Check sheet for the modelled part. Datum: model origin and axes. Units: mm. Round coordinates to 2 decimals unless told otherwise and drop trailing zeros. Loops run counter-clockwise (first coordinate to the right, second up) from the corner with the lowest first, then second, coordinate; pieces in that order, holes last. Notation, with made-up numbers: (38, 25.25) - (42, 25.25) arc R12 ccw to (42, 32.25) - close; hole circle Ø4 at (25, 80). An arc over 180 degrees is marked (long way). Answer in a Markdown table with one row per item. Add a question column.
(1) Mould release check, pull along X, two halves, no side actions. Record for faces 1 (the cylindrical face through (-1.38, 0.07, 6.2)), 2 (the flat face through (21.997, 0, 0)), 3 (the conical face through (-0.056, -4.522, -22.824)): +X half, -X half, draft (parallel to the pull), parting line (faces both ways), or undercut.
(2) Thickness scan on line 1 along Z through (x, y) = (0, -2); line 2 along Z through (x, y) = (1, 2); line 3 along X through (y, z) = (2.5, 0.5). Record the ranges inside material, lowest first.
(3) Gauge pin test, flat ends, axial feed: pin 1 (1 mm diameter, centred on x = -12.5, y = 2, fed in from +Z); pin 2 (1.5 mm diameter, centred on y = -1.5, z = 17.5, fed in from +X); pin 3 (10 mm diameter, centred on x = 0, z = 0, fed in from -Y); pin 4 (3 mm diameter, centred on x = 16.5, y = 0, fed in from +Z). Record the tip position at first contact, or that the pin passes through.
(4) Cross-section at A-A on y = 2. Enter the section's corners in (x, z), then the cut area to 3 significant figures.
from build123d import *

# Parameters (mm, degrees)
BOSS_EXTRUDE1_DEPTH = 5
SKETCH2_R           = 6.35
CUT_EXTRUDE1_DEPTH  = 11
SKETCH3_OUTSIDE_W   = 97.688
SKETCH3_OUTSIDE_H   = 104.494
SKETCH3_OUTSIDE_R   = 21.997045256
CUT_EXTRUDE2_DEPTH  = 11
CUT_EXTRUDE2_TAPER  = 60


with BuildPart() as part:
    # Sketch1 → Boss-Extrude1 (new body, symmetric)
    with BuildSketch(Plane(origin=(0, 0, 0), x_dir=(1, 0, 0), z_dir=(0, 1, 0))):
        Polygon((21.997045256, 12.7), (0, 25.4), (-21.997045256, 12.7), (-21.997045256, -12.7), (0, -25.4), (21.997045256, -12.7), align=None)
    extrude(amount=BOSS_EXTRUDE1_DEPTH, both=True)

    # Sketch2 → Cut-Extrude1 (cut, through all)
    with BuildSketch(Plane(origin=(0, 5, 0), x_dir=(1, 0, 0), z_dir=(0, 1, 0))):
        Circle(SKETCH2_R)
    extrude(amount=-CUT_EXTRUDE1_DEPTH, mode=Mode.SUBTRACT)

    # Sketch3 outside → Cut-Extrude2 (cut, through all)
    with BuildSketch(Plane(origin=(0, 5, 0), x_dir=(1, 0, 0), z_dir=(0, 1, 0))):
        Rectangle(SKETCH3_OUTSIDE_W, SKETCH3_OUTSIDE_H)
        Circle(SKETCH3_OUTSIDE_R, mode=Mode.SUBTRACT)
    cut_extrude2 = extrude(amount=-CUT_EXTRUDE2_DEPTH, taper=CUT_EXTRUDE2_TAPER, mode=Mode.SUBTRACT)

    # Mirror1: Cut-Extrude2 across plane
    add(cut_extrude2.mirror(Plane.ZX), mode=Mode.SUBTRACT)


solid = part.part
Answers:
| question | item | result |
|---|---|---|
| 1 | face 1 | undercut |
| 1 | face 2 | +X half |
| 1 | face 3 | parting line |
| 2 | line 1 | z = -25.4 to -6.35, 6.35 to 25.4 |
| 2 | line 2 | z = -24.82 to -6.27, 6.27 to 24.82 |
| 2 | line 3 | x = -22 to -6.33, 6.33 to 22 |
| 3 | pin 1 | stops at z = 18.47 |
| 3 | pin 2 | stops at x = 14.98 |
| 3 | pin 3 | passes through |
| 3 | pin 4 | stops at z = 16.74 |
| 4 | outline | (-22, -12.7) - (0, -25.4) - (22, -12.7) - (22, 12.7) - (0, 25.4) - (-22, 12.7) - close; hole circle Ø12.7 at (0, 0) |
| 4 | area | 1,550 mm^2 |
